Check sheet for the modelled part. Datum: model origin and axes. Units: mm. Round coordinates to 2 decimals unless told otherwise and drop trailing zeros. Write each loop counter-clockwise with the first axis right and the second up, starting at its lowest first coordinate (ties: lowest second). Pieces come first, ordered by that corner, then holes. Notation, with made-up numbers: (17, 8) - (27, 8) arc R17 cw to (27, 34) - close; hole circle Ø6 at (57, 64.5). An arc over 180 degrees is marked (long way). Answer as a JSON object with one key per item and string values. Group by question number.
Item 1: Sectioned sample at C-C on y = 1.2. Record the boundary of the cut face in (x, z), plus the area to 3 significant figures.
Item 2: Sectioned sample at A-A on z = 0. Record the boundary of the cut face in (x, y), plus the area to 3 significant figures.
Item 3: Thickness scan on line 1 (Z direction, x = 0, y = 0.9); line 2 (Z direction, x = 1, y = 2.3). Record the ranges inside material, lowest first.
Item 4: Sectioned sample at D-D on x = 7. Record the boundary of the cut face in (y, z).
Item 5: Sectioned sample at B-B on x = 0. Record the boundary of the cut face in (y, z).
Item 6: Release check for a two-part mould opening along Z. For faces 1 (the flat face through (0, 2.5, 4)), 2 (the cylindrical face through (-2.17, 1.23, 9.76)), 3 (the cylindrical face through (-0.38, 1.23, -5.29)) record: pulls with the +Z half, pulls with the -Z half, needs draft (parallel to the pull), parting line crosses it, or undercut.
```python
from build123d import *

# Parameters (mm, degrees)
SKETCH_1_R          = 10
SKETCH_1_R_2        = 1.75
EXTRUDE_1_DEPTH     = 2.5
SKETCH_2_R          = 3.5
CUT_EXTRUDE_1_DEPTH = 3.5


with BuildPart() as part:
    # Эскиз1 → Бобышка-Вытянуть1 (new body)
    with BuildSketch(Plane(origin=(0, 0, 0), x_dir=(1, 0, 0), z_dir=(0, 1, 0))):
        Circle(SKETCH_1_R)
        with Locations((-7, 0)):
            Circle(SKETCH_1_R_2, mode=Mode.SUBTRACT)
        with Locations((0, 7)):
            Circle(SKETCH_1_R_2, mode=Mode.SUBTRACT)
        with Locations((7, 0)):
            Circle(SKETCH_1_R_2, mode=Mode.SUBTRACT)
        with Locations((0, -7)):
            Circle(SKETCH_1_R_2, mode=Mode.SUBTRACT)
    extrude(amount=EXTRUDE_1_DEPTH)

    # Эскиз2 → Вырез-Вытянуть1 (cut, through all)
    with BuildSketch(Plane(origin=(0, 2.5, 0), x_dir=(1, 0, 0), z_dir=(0, 1, 0))):
        Circle(SKETCH_2_R)
    extrude(amount=-CUT_EXTRUDE_1_DEPTH, mode=Mode.SUBTRACT)


solid = part.part
```
Completed:
{
 "1": {"outline": "circle Ø20 at (0, 0); hole circle Ø3.5 at (-7, 0); hole circle Ø7 at (0, 0); hole circle Ø3.5 at (0, -7); hole circle Ø3.5 at (0, 7); hole circle Ø3.5 at (7, 0)", "area": "237 mm²"},
 "2": {"outline": "(-10, 0) - (-8.75, 0) - (-8.75, 2.5) - (-10, 2.5) - close; (-5.25, 0) - (-3.5, 0) - (-3.5, 2.5) - (-5.25, 2.5) - close; (3.5, 0) - (5.25, 0) - (5.25, 2.5) - (3.5, 2.5) - close; (8.75, 0) - (10, 0) - (10, 2.5) - (8.75, 2.5) - close", "area": "15.0 mm²"},
 "3": {"line 1": "-10 to -8.75, -5.25 to -3.5, 3.5 to 5.25, 8.75 to 10", "line 2": "-9.95 to -8.44, -5.56 to -3.35, 3.35 to 5.56, 8.44 to 9.95"},
 "4": {"outline": "(0, -7.14) - (2.5, -7.14) - (2.5, -1.75) - (0, -1.75) - close; (0, 1.75) - (2.5, 1.75) - (2.5, 7.14) - (0, 7.14) - close"},
 "5": {"outline": "(0, -10) - (2.5, -10) - (2.5, -8.75) - (0, -8.75) - close; (0, -5.25) - (2.5, -5.25) - (2.5, -3.5) - (0, -3.5) - close; (0, 3.5) - (2.5, 3.5) - (2.5, 5.25) - (0, 5.25) - close; (0, 8.75) - (2.5, 8.75) - (2.5, 10) - (0, 10) - close"},
 "6": {"face 1": "needs draft", "face 2": "parting line crosses it", "face 3": "undercut"}
}
